Source: three-view drawing plus pictorial views. Frame: mm from the lowest corner of the part. A direction names the side the tool comes from. Round coordinates to 2 decimals unless told otherwise and drop trailing zeros. Order: outer loops, then holes, each group sorted by start corner. A loop starts at its lowest first (then second) coordinate and runs counter-clockwise, first axis right, second up. Notation, with made-up numbers: (-12.75, -4.5) -> (2.25, -4.5) arc R36 ccw to (2.25, 31.5) -> close; hole circle Ø11 at (42, 2.25). An arc over 180 degrees is marked (long way). Answer as CSV lines item,"result". Start each with the question number.
1) Line query: L1, parallel to Z at x = 6.5, y = 17.5; L2, parallel to Z at x = 8.5, y = 2; L3, parallel to X at y = 30, z = 12.5. Output: solid intervals per line, ascending.
2) Access query for the marked faces 4, 5 and 6. Directions: +Z, -Z, +X, -X, +Y, -Y. A direction counts if a zero-diameter tool reaches every point of the face in a straight line with its end or side. Return the directions, or none.
3) Section query D-D, the plane x = 3. State how many separate pieces and enclosed holes the cut face has, and give its area (3 significant figures).
4) Mould query, pull axis X, two halves, no side actions, for the marked faces 1, 2 and 3. Classes: +X half, -X half, draft (parallel to the pull), parting line (faces both ways), or undercut.
5) First-contact query: P1, Ø4.5, axis at x = 9.74, y = 16.52, coming from the +Z side. Flat tip, straight axial feed; report the tip coordinate or a pass-through.
6) Section query B-B, the plane x = 5.5. Output: boundary loops of the cut face in (y, z).
7) Section query A-A, the plane z = 4.5. Output: boundary loops of the cut face in (x, y), and give its area (3 significant figures).
8) Section query C-C, the plane y = 5.5. Output: boundary loops of the cut face in (x, z), and give its area (3 significant figures).
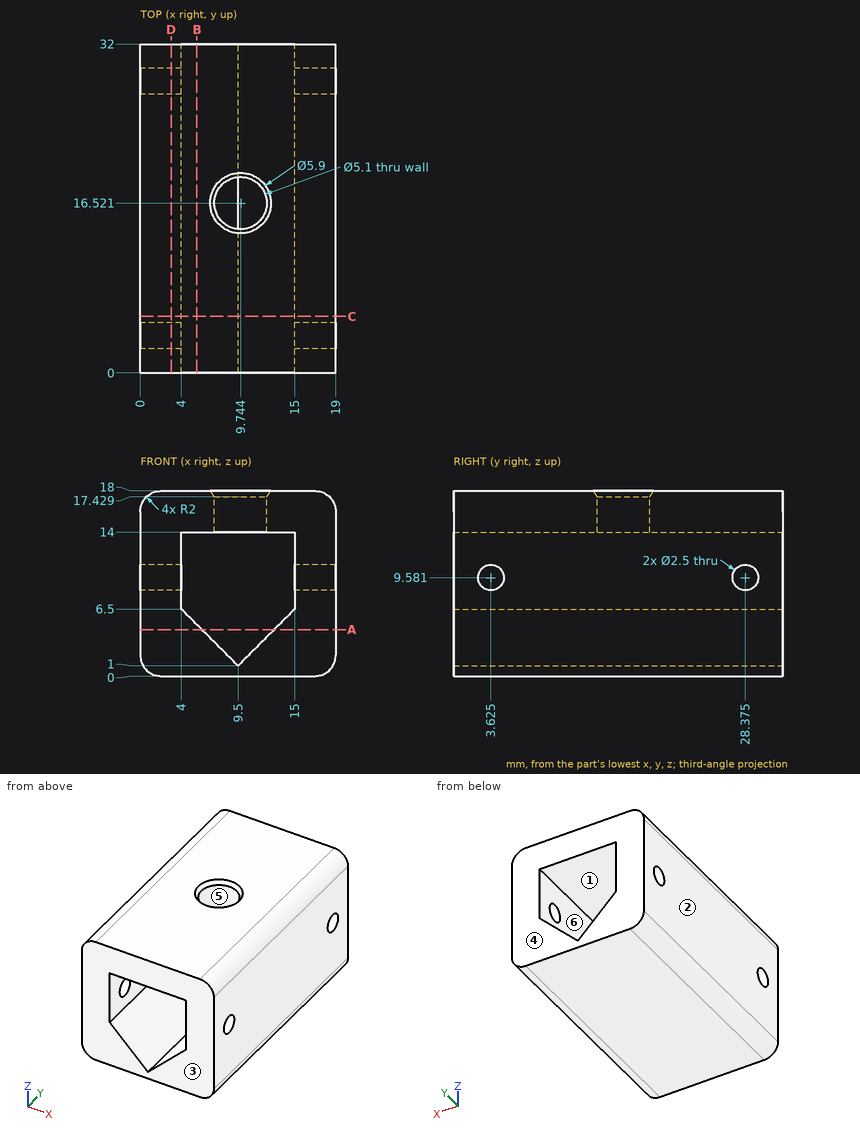
Findings:
1,L1,"z = 0 to 4, 14 to 18"
1,L2,"z = 0 to 2, 14 to 18"
1,L3,"x = 0 to 4, 15 to 19"
2,face 4,"+Z, -Z, +X, -X, +Y"
2,face 5,"+Z"
2,face 6,"+Y, -Y"
3,separate pieces,"1"
3,enclosed holes,"2"
3,area,"566 mm^2"
4,face 1,"undercut"
4,face 2,"-X half"
4,face 3,"draft"
5,P1,"stops at z = 3.49"
6,outline,"(0, 0) -> (32, 0) -> (32, 5) -> (0, 5) -> close; (0, 14) -> (32, 14) -> (32, 18) -> (0, 18) -> close"
7,outline,"(0, 0) -> (6, 0) -> (6, 32) -> (0, 32) -> close; (13, 0) -> (19, 0) -> (19, 32) -> (13, 32) -> close"
7,area,"384 mm^2"
8,outline,"(0, 2) arc R2 ccw to (2, 0) -> (17, 0) arc R2 ccw to (19, 2) -> (19, 16) arc R2 ccw to (17, 18) -> (2, 18) arc R2 ccw to (0, 16) -> close; hole (4, 6.5) -> (9.5, 1) -> (15, 6.5) -> (15, 14) -> (4, 14) -> close"
8,area,"226 mm^2"
